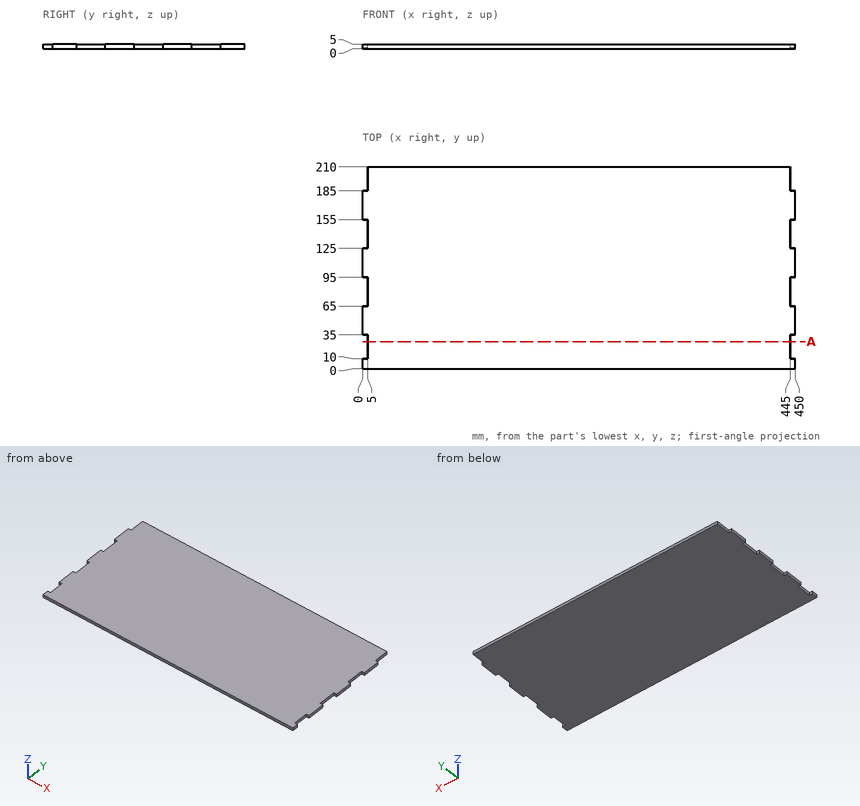
Could you check a few things on this drawing? It's one solid part, dimensions in mm from its lowest x, y, z. Coordinates: 2 decimals unless noted, no trailing zeros. Loops run counter-clockwise (first coordinate to the right, second up) from the corner with the lowest first, then second, coordinate; pieces in that order, holes last. Notation, with made-up numbers: (36.25, 59) - (76.25, 59) arc R17 ccw to (76.25, 83) - close; hole circle Ø8 at (33.25, 18). An arc over 180 degrees is marked (long way). Return JSON: item names as keys, results as strings. Group by question number.
Item 1: If we section it at A-A on y = 28: Write out the boundary of the cut face in (x, z), and give its area (3 significant figures).
Item 2: I need wall thicknesses on line 1 (X direction, y = 79.5, z = 2.55). Which ranges of the line are inside material? Lowest first, please. Write a range as from..to.
Item 3: Will these pins go through, and if not, where does the flat tip stop? P1, Ø2.5, axis at y = 196.5, z = 2.5, coming from the +X side; P2, Ø2.5, axis at y = 23.5, z = 3, coming from the -X side; P3, Ø1.5, axis at x = 2.5, z = 1.5, coming from the +Y side.
Calculated:
{
 "1": {"outline": "(5, 0) - (445, 0) - (445, 5) - (5, 5) - close", "area": "2,200 mm^2"},
 "2": {"line 1": "x = 5..445"},
 "3": {"P1": "stops at x = 445", "P2": "stops at x = 5", "P3": "stops at y = 185"}
}
